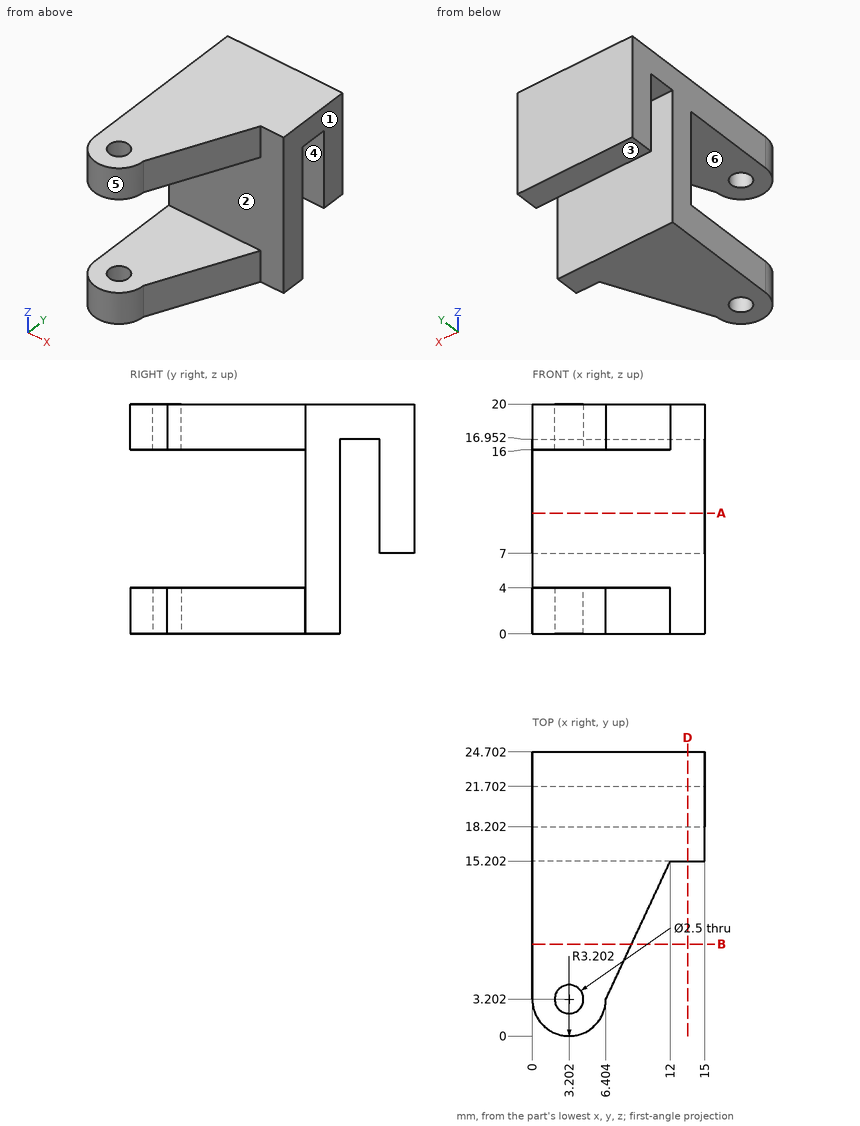
Could you check a few things on this drawing? It's one solid part, dimensions in mm from its lowest x, y, z. A direction names the side the tool comes from. Coordinates: 2 decimals unless noted, no trailing zeros. Order: outer loops, then holes, each group sorted by start corner. A loop starts at its lowest first (then second) coordinate and runs counter-clockwise, first axis right, second up. Notation, with made-up numbers: (42, -38.75) - (91, -38.75) arc R24 cw to (91, -24.75) - close; hole circle Ø8 at (60.25, 66). An arc over 180 degrees is marked (long way). One line per question, with ' | ' between items. Start each with the question number.
1. If we mould it in two halves opening along Z, with no side actions, what happens to the marked faces 1, 2 and 3? For each: released by +Z, released by -Z, zero draft, split by the parting line, or undercut.
2. If we section it at B-B (y = 8): Write out the boundary of the cut face in (x, z).
3. If we section it at A-A (z = 10.5): Write out the boundary of the cut face in (x, y).
4. Please list where these lines run through material, in increasing order: line 1 along Z through (x, y) = (6, 12); line 2 along Y through (x, z) = (10.5, 11); line 3 along Y through (x, z) = (13, 19). Write a range as [from, to].
5. If we section it at D-D (x = 13.5): Write out the boundary of the cut face in (y, z).
6. I'm going to push flat-ended pins straight in: pin 1 Ø1.5 at (x, y) = (4, 23.5) entering from -Z; pin 2 Ø1 at (x, z) = (5.5, 5) entering from -Y; pin 3 Ø1 at (y, z) = (11.5, 16) entering from +X. Where does each tip first touch, or does it pass through?
7. Which directions (+Z, -Z, +X, -X, +Y, -Y) give clear straight access to the entire face, cutting with the end or side of a thin tool? Please do the marked faces 4, 5 and 6.
Model answer:
1) face 1: zero draft | face 2: undercut | face 3: released by -Z
2) outline: (0, 0) - (8.64, 0) - (8.64, 4) - (0, 4) - close; (0, 16) - (8.64, 16) - (8.64, 20) - (0, 20) - close
3) outline: (0, 15.2) - (15, 15.2) - (15, 18.2) - (0, 18.2) - close; (0, 21.7) - (15, 21.7) - (15, 24.7) - (0, 24.7) - close
4) line 1: z = [0, 4], [16, 20] | line 2: y = [15.2, 18.2], [21.7, 24.7] | line 3: y = [15.2, 24.7]
5) outline: (15.2, 0) - (18.2, 0) - (18.2, 16.95) - (21.7, 16.95) - (21.7, 7) - (24.7, 7) - (24.7, 20) - (15.2, 20) - close
6) pin 1: stops at z = 7 | pin 2: stops at y = 15.2 | pin 3: stops at x = 10.51
7) face 4: -Z, +X, -X | face 5: +Z, -Z, -Y | face 6: +X, -X, -Y
